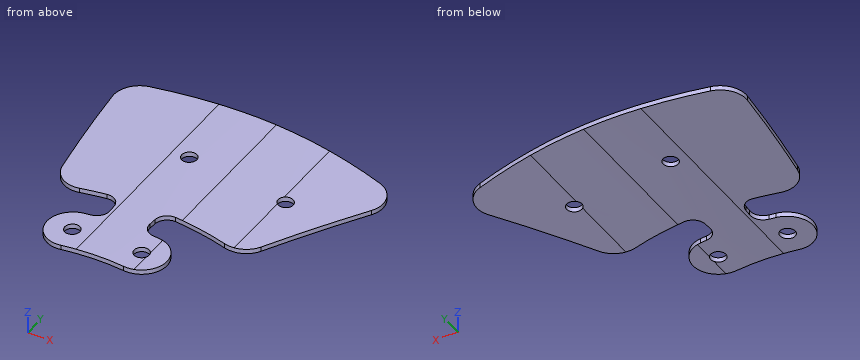
```python
from build123d import *

# Parameters (mm, degrees)
SKETCH9_W               = 63
SKETCH9_H               = 97
BOSS_EXTRUDE3_DEPTH     = 0.9
FLEX1_DEPTH             = 97
FLEX1_2_DEPTH           = 97
HOLES_DEPTH             = 105.800393682
HOLES_DEPTH_BACK        = 105.800393682
SKETCH10_R              = 1.5
CUT_EXTRUDE2_DEPTH      = 105.800393775
CUT_EXTRUDE2_DEPTH_BACK = 105.800393775
SKETCH11_W              = 63.006108503
SKETCH11_H              = 97
FILLET1_START           = -0.513450093
FILLET1_DEPTH           = 1.413450171
FILLET2_R               = 2.5


with BuildPart() as part:
    # Sketch9 → Boss-Extrude3 (new body)
    with BuildSketch(Plane.XY):
        with Locations((8.161949416, 48.5)):
            Rectangle(SKETCH9_W, SKETCH9_H)
    extrude(amount=BOSS_EXTRUDE3_DEPTH)

    # Flex1: read off the stored shape, not the designer's step
    # Flex1 outline → Flex1 (cut)
    with BuildSketch(Plane(origin=(0, 0, 0), x_dir=(1, 0, 0), z_dir=(0, 1, 0))):
        Polygon((39.661949416, 0), (39.657624847, 0), (39.661949416, -0.1981922), align=None)
        Polygon((-23.338050584, -0.198192162), (-23.333726016, 0), (-23.338050584, 0), align=None)
        with BuildLine():
            Line((39.661949416, -0.9), (39.661949416, -0.33823319))
            Line((39.661949416, -0.33823319), (19.669763126, -0.774464246))
            ThreePointArc((19.669763126, -0.774464246), (13.91619862, -0.868615128), (8.161949416, -0.9))
            Line((8.161949416, -0.9), (39.661949416, -0.9))
        make_face()
        with BuildLine():
            Line((-3.345864294, -0.774464246), (-23.338050584, -0.33823319))
            Line((-23.338050584, -0.33823319), (-23.338050584, -0.9))
            Line((-23.338050584, -0.9), (8.161949416, -0.9))
            ThreePointArc((8.161949416, -0.9), (2.407700212, -0.868615128), (-3.345864294, -0.774464246))
        make_face()
    extrude(amount=FLEX1_DEPTH, mode=Mode.SUBTRACT)

    # Flex1 2 outline → Flex1 2 (add)
    with BuildSketch(Plane(origin=(0, 0, 0), x_dir=(1, 0, 0), z_dir=(0, 1, 0))):
        with BuildLine():
            ThreePointArc((8.161950743, 0), (2.417518157, 0.031331319), (-3.326230898, 0.125321578))
            Line((-3.326230898, 0.125321578), (-23.321471439, 0.561619279))
            Line((-23.321471439, 0.561619279), (-23.333726016, 0))
            Line((-23.333726016, 0), (8.161950743, 0))
        make_face()
        with BuildLine():
            ThreePointArc((19.650129729, 0.125321578), (13.906382001, 0.031331334), (8.161950743, 0))
            Line((8.161950743, 0), (39.657624847, 0))
            Line((39.657624847, 0), (39.645370271, 0.561619279))
            Line((39.645370271, 0.561619279), (19.650129729, 0.125321578))
        make_face()
        Polygon((39.665003667, -0.338166546), (39.661949416, -0.1981922), (39.661949416, -0.33823319), align=None)
        Polygon((-23.338050584, -0.33823319), (-23.338050584, -0.198192162), (-23.341104836, -0.338166546), align=None)
    extrude(amount=FLEX1_2_DEPTH)

    # Sketch10 → Holes (cut, two sides: drawn at the far end of the back side and taken through both)
    with BuildSketch(Plane.XY.offset(-HOLES_DEPTH_BACK)):
        with Locations(Location((0, 79.75, 0), (0, 0, 180))):
            Circle(SKETCH10_R)
        with Locations(Location((20.640818847, 77.032584647, 0), (0, 0, 228.665080439))):
            Circle(SKETCH10_R)
        with Locations(Location((-6.852625092, 52.050855222, 0), (0, 0, 180))):
            Circle(SKETCH10_R)
        with Locations(Location((6.852625092, 52.050855222, 0), (0, 0, 180))):
            Circle(SKETCH10_R)
    extrude(amount=HOLES_DEPTH + HOLES_DEPTH_BACK, mode=Mode.SUBTRACT)

    # Sketch11 → Cut-Extrude2 (cut, two sides: drawn at the far end of the back side and taken through both)
    with BuildSketch(Plane.XY.offset(-CUT_EXTRUDE2_DEPTH_BACK)):
        with Locations((8.161949415, 48.5)):
            Rectangle(SKETCH11_W, SKETCH11_H)
        with BuildLine():
            Line((4.185800271, 63.862971087), (3.760679931, 57.376888086))
            ThreePointArc((3.760679931, 57.376888086), (5.635985569, 57.223121784), (7.505256053, 57.008079529))
            ThreePointArc((7.505256053, 57.008079529), (11.809849398, 51.398224261), (6.19999413, 47.093630915))
            ThreePointArc((6.19999413, 47.093630915), (0, 47.5), (-6.19999413, 47.093630915))
            ThreePointArc((-6.19999413, 47.093630915), (-11.809849398, 51.398224261), (-7.505256053, 57.008079529))
            ThreePointArc((-7.505256053, 57.008079529), (-5.635985569, 57.223121784), (-3.760679931, 57.376888086))
            Line((-3.760679931, 57.376888086), (-4.185800271, 63.862971087))
            ThreePointArc((-4.185800271, 63.862971087), (-10.501653038, 63.132521599), (-16.713864661, 61.779015273))
            ThreePointArc((-16.713864661, 61.779015273), (-19.180957256, 77.436335693), (-20.828588873, 93.200965046))
            ThreePointArc((-20.828588873, 93.200965046), (8.724041697, 95.100689253), (37.437803154, 87.855909847))
            ThreePointArc((37.437803154, 87.855909847), (29.127303266, 74.268784811), (21.532663784, 60.268933874))
            ThreePointArc((21.532663784, 60.268933874), (12.984187468, 62.669058361), (4.185800271, 63.862971087))
        make_face(mode=Mode.SUBTRACT)
    extrude(amount=CUT_EXTRUDE2_DEPTH + CUT_EXTRUDE2_DEPTH_BACK, mode=Mode.SUBTRACT)

    # Fillet1: read off the stored shape, not the designer's step
    # Fillet1 outline → Fillet1 (cut)
    with BuildSketch(Plane.XY.offset(FILLET1_START)):
        with BuildLine():
            ThreePointArc((-16.713864661, 61.779015273), (-14.256840633, 62.391846384), (-11.777496683, 62.906999387))
            ThreePointArc((-11.777496683, 62.906999387), (-15.563592629, 63.724516542), (-17.629773662, 67.000757185))
            ThreePointArc((-17.629773662, 67.000757185), (-17.183202347, 64.387889585), (-16.713864661, 61.779015273))
        make_face()
        with BuildLine():
            ThreePointArc((21.532663784, 60.268933874), (22.490522566, 62.133675811), (23.461092679, 63.991833391))
            ThreePointArc((23.461092679, 63.991833391), (20.999228882, 61.722888632), (17.657666024, 61.515907135))
            ThreePointArc((17.657666024, 61.515907135), (19.605081566, 60.923236756), (21.532663784, 60.268933874))
        make_face()
        with BuildLine():
            ThreePointArc((37.437803154, 87.855909847), (34.544505688, 89.033292238), (31.614250404, 90.115421385))
            ThreePointArc((31.614250404, 90.115421385), (34.674360622, 87.060431172), (34.20794214, 82.761629764))
            ThreePointArc((34.20794214, 82.761629764), (35.810360655, 85.316702623), (37.437803154, 87.855909847))
        make_face()
        with BuildLine():
            ThreePointArc((-20.828588873, 93.200965046), (-20.644293019, 90.952269753), (-20.443312617, 88.705004224))
            ThreePointArc((-20.443312617, 88.705004224), (-19.435950656, 92.207056404), (-16.319289437, 94.095328217))
            ThreePointArc((-16.319289437, 94.095328217), (-18.579321492, 93.675283895), (-20.828588873, 93.200965046))
        make_face()
    extrude(amount=FILLET1_DEPTH, mode=Mode.SUBTRACT)

    # Fillet2
    fillet2_edges = [part.edges().sort_by_distance(p)[0] for p in [
        (3.760679931, 57.376888086, 0.431623426),
        (-3.760679931, 57.376888086, 0.315305823),
        (4.185800271, 63.862971087, 0.435002027),
        (-4.185800271, 63.862971087, 0.306029665),
    ]]
    fillet(fillet2_edges, radius=FILLET2_R)


solid = part.part
```
Read the model definition and answer for the solid it produces. Units are mm, in the model's axes. Give positions to 0.01 mm unless a question says otherwise; leave off trailing zeros. Write each loop counter-clockwise with the first axis right and the second up, starting at its lowest first coordinate (ties: lowest second). Pieces come first, ordered by that corner, then holes. Notation, with made-up numbers: (-32.75, 1) - (20.25, 1) arc R12 cw to (20.25, 7) - close; hole circle Ø4 at (42, 63). An arc over 180 degrees is marked (long way). Write item = value, one per line. Start each with the question number.
Item 1: Find the intervals of material crossed by probe 1 along X at (y, z) = (52, 0.45); probe 2 along Y at (x, z) = (0, 0.3); probe 3 along X at (y, z) = (79.75, 0.2), in increasing order. Write a range as [from, to].
Item 2: Each of these flat-tipped pins is pushed along its axis until it touches: P1, Ø1.8, axis at x = 20.64, y = 77.03, coming from the +Z side; P2, Ø6, axis at x = -13, y = 84, coming from the -Z side; P3, Ø2, axis at x = 20, y = 75.5, coming from the +Z side; P4, Ø4, axis at x = -6.85, y = 52.05, coming from the -Z side. Where does it stop, or does it pass through?
Item 3: Find section A-A (y = 79.75). Give the vertices of the cut face in (x, z).
Item 4: Find section B-B (x = 0). Give the vertices of the cut face in (y, z), then the cut area to 3 significant figures.
Item 5: Find section C-C (y = 68.5). Give the vertices of the cut face in (x, z).
Item 6: Find section D-D (x = -11). Give the vertices of the cut face in (y, z), then the cut area to 3 significant figures.
Response:
q1.probe_1 = [-11.85, -8.35], [-5.35, 5.35], [8.35, 11.85]
q1.probe_2 = [47.5, 78.25], [81.25, 95.5]
q1.probe_3 = [-19.47, -1.5], [1.5, 32.36]
q2.P1 = through
q2.P2 = -0.4
q2.P3 = 0.79
q2.P4 = -0.25
q3.outline = (-19.47, -0.48) - (-3.33, -0.13) arc R526.62 cw to (-1.5, -0.09) - (-1.5, 0.81) arc R527.52 ccw to (-3.35, 0.77) - (-19.47, 0.42) - close; (1.5, -0.04) arc R526.62 cw to (8.16, 0) arc R526.62 cw to (19.65, -0.13) - (32.36, -0.4) - (32.36, 0.5) - (19.67, 0.77) arc R527.52 ccw to (1.5, 0.86) - close
q4.outline = (47.5, -0.06) - (78.25, -0.06) - (78.25, 0.84) - (47.5, 0.84) - close; (81.25, -0.06) - (95.5, -0.06) - (95.5, 0.84) - (81.25, 0.84) - close
q4.area = 40.5 mm²
q5.outline = (-17.88, -0.44) - (-3.33, -0.13) arc R526.62 cw to (8.16, 0) arc R526.62 cw to (19.65, -0.13) - (25.88, -0.26) - (25.88, 0.64) - (19.67, 0.77) arc R527.52 ccw to (-3.35, 0.77) - (-17.88, 0.46) - close
q6.outline = (49.26, -0.29) - (54.84, -0.29) - (54.84, 0.61) - (49.26, 0.61) - close; (63.05, -0.29) - (94.86, -0.29) - (94.86, 0.61) - (63.05, 0.61) - close
q6.area = 33.7 mm²
